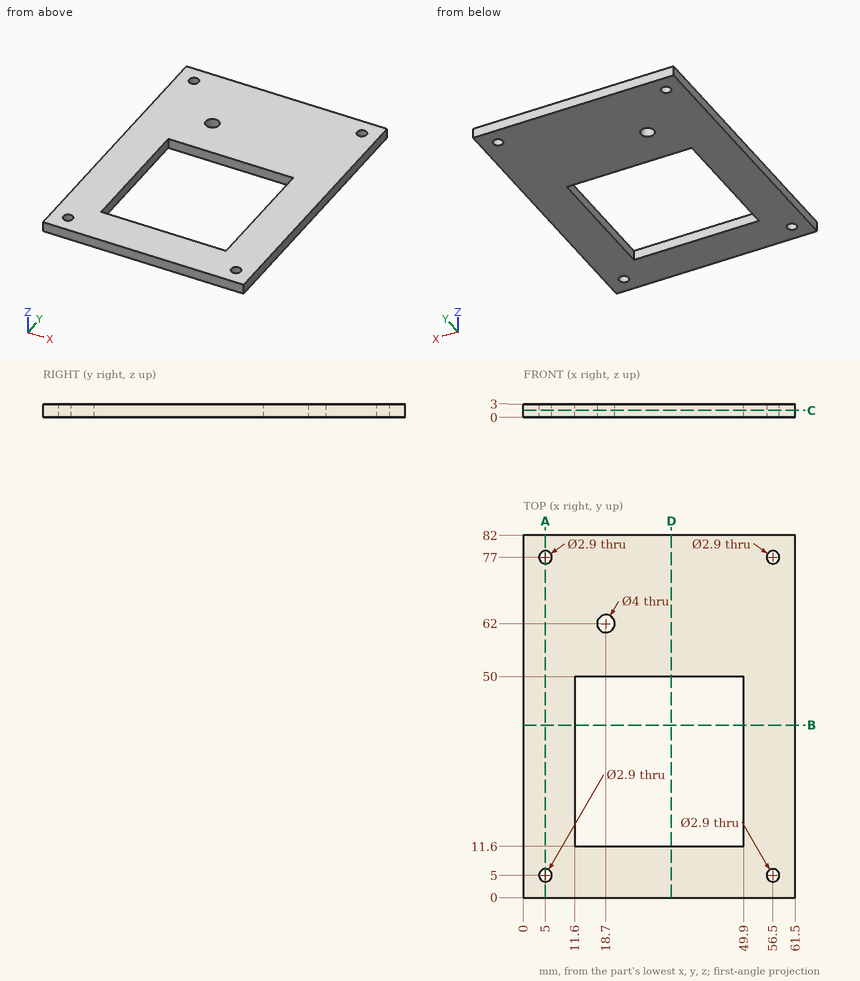
Check sheet for the drawn part. Datum: minimum x, y, z corner. Units: mm. Give positions to 0.01 mm unless a question says otherwise; leave off trailing zeros. Order: outer loops, then holes, each group sorted by start corner. A loop starts at its lowest first (then second) coordinate and runs counter-clockwise, first axis right, second up. Notation, with made-up numbers: (-29, 81) -> (27, 81) arc R12 ccw to (27, 103) -> close; hole circle Ø4 at (23, -21). An arc over 180 degrees is marked (long way). Use a Markdown table: item, result.
1) Section check D-D, the plane x = 33.5. Record the boundary of the cut face in (y, z).
Results:
| item | result |
|---|---|
| outline | (0, 0) -> (11.6, 0) -> (11.6, 3) -> (0, 3) -> close; (50, 0) -> (82, 0) -> (82, 3) -> (50, 3) -> close |
2) Material ranges on probe 1 along Y at (x, z) = (56.5, 1.1); probe 2 along X at (y, z) = (77, 0.9); probe 3 along Y at (x, z) = (37, 0.6), recorded low to high.
Results:
| item | result |
|---|---|
| probe 1 | 0 to 3.55, 6.45 to 75.55, 78.45 to 82 |
| probe 2 | 0 to 3.55, 6.45 to 55.05, 57.95 to 61.5 |
| probe 3 | 0 to 11.6, 50 to 82 |
3) Section check A-A, the plane x = 5. Record the boundary of the cut face in (y, z).
Results:
| item | result |
|---|---|
| outline | (0, 0) -> (3.55, 0) -> (3.55, 3) -> (0, 3) -> close; (6.45, 0) -> (75.55, 0) -> (75.55, 3) -> (6.45, 3) -> close; (78.45, 0) -> (82, 0) -> (82, 3) -> (78.45, 3) -> close |
4) Section check B-B, the plane y = 39. Record the boundary of the cut face in (x, z).
Results:
| item | result |
|---|---|
| outline | (0, 0) -> (11.6, 0) -> (11.6, 3) -> (0, 3) -> close; (49.9, 0) -> (61.5, 0) -> (61.5, 3) -> (49.9, 3) -> close |
5) Section check C-C, the plane z = 1.55. Record the boundary of the cut face in (x, y), then the cut area to 3 significant figures.
Results:
| item | result |
|---|---|
| outline | (0, 0) -> (61.5, 0) -> (61.5, 82) -> (0, 82) -> close; hole circle Ø2.9 at (5, 5); hole circle Ø2.9 at (5, 77); hole (11.6, 11.6) -> (49.9, 11.6) -> (49.9, 50) -> (11.6, 50) -> close; hole circle Ø4 at (18.7, 62); hole circle Ø2.9 at (56.5, 5); hole circle Ø2.9 at (56.5, 77) |
| area | 3,530 mm² |
6) Depth check by flat-ended pin: pin 1 Ø6 at (x, y) = (11.5, 60.5) entering from -Z. Enter the tip coordinate at first touch or a pass-through.
Results:
| item | result |
|---|---|
| pin 1 | z = 0 |
